Read the model definition and answer for the solid it produces. Units are mm, in the model's axes. A direction names the side the tool comes from. Round coordinates to 2 decimals unless told otherwise and drop trailing zeros. Write each loop counter-clockwise with the first axis right and the second up, starting at its lowest first coordinate (ties: lowest second). Pieces come first, ordered by that corner, then holes. Notation, with made-up numbers: (72, 2.25) - (128, 2.25) arc R12 cw to (128, 25.25) - close; hole circle Ø4 at (68, 39). An arc over 180 degrees is marked (long way). Use one line per item in the form item = value. Start each with the question number.
1) The part is cut by section C-C, the plane x = -14. Give the vertices of the cut face in (y, z).
2) The part is cut by section B-B, the plane y = 16. Give the vertices of the cut face in (x, z), plus the area to 3 significant figures.
3) The part is cut by section D-D, the plane x = -1. Give the vertices of the cut face in (y, z).
4) Each of these flat-tipped pins is pushed along its axis until it touches: pin 1 (2.5 mm diameter, centred on y = 20, z = -8, fed in from -X); pin 2 (5 mm diameter, centred on x = -15.5, z = 10, fed in from +Y); pin 3 (1.5 mm diameter, centred on y = 13, z = -6, fed in from +X). Where does it stop, or does it pass through?
5) The part is cut by section A-A, the plane z = -0.75. Give the vertices of the cut face in (x, y).
6) For faces 4 (the face through (-2.4, 14.3, 3.12)), 5 (the face through (-10.052, 14, -6)), 6 (the face through (-8.052, 19, -8)), 7 (the face through (9.948, 14, -6)), 8 (the face through (-13.054, 1.479, -5.718)), determine the directions among +Z, -Z, +X, -X, +Y, -Y from which every point of the face is accessible in a straight line to the end or side of a thin tool.
7) Consider line 1 along Z through (x, y) = (7, 24.5); line 2 along Z through (x, y) = (8, 21.75); line 3 along X through (y, z) = (7.25, 1). Determine where each line is inside the solid, lowest interval first. Write a range as from..to.
8) For a pull along X with two mould halves and no side action, classify faces 1 (the face through (0, 1, 14.37)), 2 (the face through (19.948, 1, 0)), 3 (the face through (16.796, 1.479, -6.396)) as released by +X, released by -X, zero draft, split by the parting line, or undercut.
from build123d import *

# Parameters (mm, degrees)
ESQUISSE3_W             = 10
ESQUISSE3_H             = 15
ESQUISSE3_H_2           = 10
ESQUISSE3_H_3           = 5
BOSS_EXTRU_1_DEPTH      = 3
ESQUISSE4_W             = 10
ESQUISSE4_H             = 5
ESQUISSE4_H_2           = 3.75
BOSS_EXTRU_2_DEPTH      = 17
ENL_V_MAT_EXTRU_1_DEPTH = 5
ENL_V_MAT_EXTRU_2_DEPTH = 18.75
ESQUISSE8_W             = 20
ESQUISSE8_H             = 18.75
ESQUISSE8_W_2           = 16
ESQUISSE8_H_2           = 5
BOSS_EXTRU_3_DEPTH      = 6


with BuildPart() as part:
    # Esquisse3 → Boss.-Extru.1 (new body)
    with BuildSketch(Plane(origin=(0, 0, 0), x_dir=(1, 0, 0), z_dir=(0, 1, 0))):
        with Locations((-15.05164944, -6.870348765)):
            Rectangle(ESQUISSE3_W, ESQUISSE3_H)
        with Locations((14.94835056, -6.870348765)):
            Rectangle(ESQUISSE3_W, ESQUISSE3_H)
        with BuildLine():
            Line((-10.05164944, 5.629651235), (-10.05164944, 15.629651235))
            Line((-10.05164944, 15.629651235), (-20.05164944, 15.629651235))
            Line((-20.05164944, 15.629651235), (-20.05164944, 5.629651235))
            Line((-20.05164944, 5.629651235), (-17.05164944, 5.629651235))
            ThreePointArc((-17.05164944, 5.629651235), (-15.05164944, 7.629651235), (-13.05164944, 5.629651235))
            Line((-13.05164944, 5.629651235), (-10.05164944, 5.629651235))
        make_face()
        with BuildLine():
            Line((-10.05164944, 0.629651235), (-10.05164944, 5.629651235))
            Line((-10.05164944, 5.629651235), (-13.05164944, 5.629651235))
            ThreePointArc((-13.05164944, 5.629651235), (-15.05164944, 3.629651235), (-17.05164944, 5.629651235))
            Line((-17.05164944, 5.629651235), (-20.05164944, 5.629651235))
            Line((-20.05164944, 5.629651235), (-20.05164944, 0.629651235))
            Line((-20.05164944, 0.629651235), (-10.05164944, 0.629651235))
        make_face()
        with Locations((-5.05164944, 10.629651235)):
            Rectangle(ESQUISSE3_W, ESQUISSE3_H_2)
        with Locations((4.94835056, 10.629651235)):
            Rectangle(ESQUISSE3_W, ESQUISSE3_H_2)
        with BuildLine():
            Line((19.94835056, 15.629651235), (9.94835056, 15.629651235))
            Line((9.94835056, 15.629651235), (9.94835056, 5.629651235))
            Line((9.94835056, 5.629651235), (12.94835056, 5.629651235))
            ThreePointArc((12.94835056, 5.629651235), (14.94835056, 7.629651235), (16.94835056, 5.629651235))
            Line((16.94835056, 5.629651235), (19.94835056, 5.629651235))
            Line((19.94835056, 5.629651235), (19.94835056, 15.629651235))
        make_face()
        with BuildLine():
            Line((12.94835056, 5.629651235), (9.94835056, 5.629651235))
            Line((9.94835056, 5.629651235), (9.94835056, 0.629651235))
            Line((9.94835056, 0.629651235), (19.94835056, 0.629651235))
            Line((19.94835056, 0.629651235), (19.94835056, 5.629651235))
            Line((19.94835056, 5.629651235), (16.94835056, 5.629651235))
            ThreePointArc((16.94835056, 5.629651235), (14.94835056, 3.629651235), (12.94835056, 5.629651235))
        make_face()
        with Locations((4.94835056, -6.870348765)):
            Rectangle(ESQUISSE3_W, ESQUISSE3_H)
        with Locations((-5.05164944, -6.870348765)):
            Rectangle(ESQUISSE3_W, ESQUISSE3_H)
        with Locations((4.94835056, 3.129651235)):
            Rectangle(ESQUISSE3_W, ESQUISSE3_H_3)
        with Locations((-5.05164944, 3.129651235)):
            Rectangle(ESQUISSE3_W, ESQUISSE3_H_3)
    extrude(amount=BOSS_EXTRU_1_DEPTH)

    # Esquisse4 → Boss.-Extru.2 (add)
    with BuildSketch(Plane(origin=(0, 3, 0), x_dir=(1, 0, 0), z_dir=(0, 1, 0))):
        with Locations((-5.05164944, 3.129651235)):
            Rectangle(ESQUISSE4_W, ESQUISSE4_H)
        with Locations((-5.05164944, -1.245348765)):
            Rectangle(ESQUISSE4_W, ESQUISSE4_H_2)
        with Locations((4.94835056, -1.245348765)):
            Rectangle(ESQUISSE4_W, ESQUISSE4_H_2)
        with Locations((4.94835056, 3.129651235)):
            Rectangle(ESQUISSE4_W, ESQUISSE4_H)
        Polygon((-0.05164944, 15.629651235), (-0.05164944, 5.629651235), (9.94835056, 5.629651235), (9.94835056, 8.129651235), align=None)
        Polygon((-10.05164944, 8.129651235), (-10.05164944, 5.629651235), (-0.05164944, 5.629651235), (-0.05164944, 15.629651235), align=None)
        Polygon((-10.05164944, 15.629651235), (-10.05164944, 8.129651235), (-0.05164944, 15.629651235), align=None)
        Polygon((9.94835056, 15.629651235), (-0.05164944, 15.629651235), (9.94835056, 8.129651235), align=None)
    extrude(amount=BOSS_EXTRU_2_DEPTH)

    # Esquisse6 → Enlèv. mat.-Extru.1 (cut)
    with BuildSketch(Plane(origin=(0, 0, -10.629651235), x_dir=(-1, 0, 0), z_dir=(0, 0, -1))):
        with BuildLine():
            Line((8.05164944, 20), (-7.94835056, 20))
            Line((-7.94835056, 20), (-7.94835056, 12))
            ThreePointArc((-7.94835056, 12), (0.05164944, 4), (8.05164944, 12))
            Line((8.05164944, 12), (8.05164944, 20))
        make_face()
    extrude(amount=-ENL_V_MAT_EXTRU_1_DEPTH, mode=Mode.SUBTRACT)

    # Esquisse7 → Enlèv. mat.-Extru.2 (cut)
    with BuildSketch(Plane(origin=(0, 0, -15.629651235), x_dir=(-1, 0, 0), z_dir=(0, 0, -1))):
        with BuildLine():
            ThreePointArc((3.05164944, 12), (2.823288037, 13.148050297), (2.172969783, 14.121320344))
            Line((2.172969783, 14.121320344), (0.05164944, 12))
            Line((0.05164944, 12), (2.172969783, 9.878679656))
            ThreePointArc((2.172969783, 9.878679656), (2.823288037, 10.851949703), (3.05164944, 12))
        make_face()
        with BuildLine():
            Line((0.05164944, 12), (2.172969783, 14.121320344))
            ThreePointArc((2.172969783, 14.121320344), (0.05164944, 15), (-2.069670904, 14.121320344))
            Line((-2.069670904, 14.121320344), (0.05164944, 12))
        make_face()
        with BuildLine():
            ThreePointArc((-2.069670904, 9.878679656), (0.05164944, 9), (2.172969783, 9.878679656))
            Line((2.172969783, 9.878679656), (0.05164944, 12))
            Line((0.05164944, 12), (-2.069670904, 9.878679656))
        make_face()
        with BuildLine():
            Line((0.05164944, 12), (-2.069670904, 14.121320344))
            ThreePointArc((-2.069670904, 14.121320344), (-2.94835056, 12), (-2.069670904, 9.878679656))
            Line((-2.069670904, 9.878679656), (0.05164944, 12))
        make_face()
    extrude(amount=-ENL_V_MAT_EXTRU_2_DEPTH, mode=Mode.SUBTRACT)

    # Esquisse8 → Boss.-Extru.3 (add)
    with BuildSketch(Plane(origin=(0, 20, 0), x_dir=(1, 0, 0), z_dir=(0, 1, 0))):
        with Locations((-0.05164944, 6.254651235)):
            Rectangle(ESQUISSE8_W, ESQUISSE8_H)
        with Locations((-0.05164944, 8.129651235)):
            Rectangle(ESQUISSE8_W_2, ESQUISSE8_H_2, mode=Mode.SUBTRACT)
    extrude(amount=BOSS_EXTRU_3_DEPTH)


solid = part.part
Geometry results:
q1.outline = (0, -15.63) - (3, -15.63) - (3, -7.33) - (0, -7.33) - close; (0, -3.93) - (3, -3.93) - (3, 14.37) - (0, 14.37) - close
q2.outline = (-10.05, -15.63) - (9.95, -15.63) - (9.95, 3.12) - (-10.05, 3.12) - close; hole (-8.05, -10.63) - (7.95, -10.63) - (7.95, -5.63) - (-8.05, -5.63) - close
q2.area = 295 mm2
q3.outline = (0, -15.63) - (9.15, -15.63) - (9.15, -10.63) - (4.06, -10.63) - (4.06, -5.63) - (9.15, -5.63) - (9.15, 3.12) - (3, 3.12) - (3, 14.37) - (0, 14.37) - close; (14.85, -15.63) - (26, -15.63) - (26, -10.63) - (14.85, -10.63) - close; (14.85, -5.63) - (26, -5.63) - (26, 3.12) - (14.85, 3.12) - close
q4.pin_1 = -10.05
q4.pin_2 = 3
q4.pin_3 = 9.95
q5.outline = (-20.05, 0) - (19.95, 0) - (19.95, 3) - (9.95, 3) - (9.95, 26) - (-10.05, 26) - (-10.05, 3) - (-20.05, 3) - close; hole circle Ø6 at (-0.05, 12)
q6.face_4 = +Z, +X, -X, +Y
q6.face_5 = +Z, -Z, -X, +Y
q6.face_6 = +Y
q6.face_7 = +Z, -Z, +X, +Y
q6.face_8 = +Y, -Y
q7.line_1 = -15.63..-10.63, -5.63..3.12
q7.line_2 = -15.63..3.12
q7.line_3 = -10.05..9.95
q8.face_1 = zero draft
q8.face_2 = released by +X
q8.face_3 = undercut
